Autodesk Inventor part; units mm, degrees
ref_plane "YZ Plane" through (0, 0, 0) normal (1, 0, 0) x (0, 1, 0)
ref_plane "XZ Plane" through (0, 0, 0) normal (0, 1, 0) x (-1, 0, 0)
ref_plane "XY Plane" through (0, 0, 0) normal (0, 0, 1) x (1, 0, 0)
sketch "Sketch1" plane through (0, 0, 0) normal (0, 0, 1) x (1, 0, 0)
  line L0 (0, 0) -> (24.765, 0)
  line L1 (24.765, 0) -> (24.765, 5.3594)
  line L2 (24.765, 5.3594) -> (0, 5.3594)
  line L3 (0, 5.3594) -> (0, 0)
  line L4 (23.7236, 7.3152) -> (30.734, 7.3152)
  line L5 (30.734, 7.3152) -> (30.734, 14.3256)
  line L6 (30.734, 14.3256) -> (23.7236, 14.3256)
  line L7 (23.7236, 14.3256) -> (23.7236, 7.3152)
  arc A0 (23.7236, 8.9916) -> (17.4244, 5.3594) centre (23.7236, 1.7133) ccw
  line L8 (24.765, 5.3594) -> (24.765, 7.3152)
  dimension "d0" = 24.765
  dimension "d1" = 5.3594
  dimension "d2" = 30.734
  dimension "d3" = 7.0104
  dimension "d4" = 14.3256
  dimension "d5" = 17.4244
  dimension "d6" = 5.334
extrude "Extrusion1" add sketch "Sketch1" along normal blind 25.4
fillet "Fillet1" radius 1.27 1 edges at (30.734, 14.3256, 12.7)
fillet "Fillet2" radius 1.27 2 edges at (30.734, 7.3152, 12.7) (23.7236, 14.3256, 12.7)
fillet "Fillet3" radius 1.27 5 edges at (23.7236, 8.9916, 12.7) (24.765, 7.3152, 12.7) (24.765, 0, 12.7) (0, 0, 12.7) (0, 5.3594, 12.7)
properties part number "Igus Slider"
The listing builds one solid part. Answer for the finished solid, in the listing's coordinates (mm). A direction names the side the tool comes from. Coordinates: 2 decimals unless noted, no trailing zeros. Loops run counter-clockwise (first coordinate to the right, second up) from the corner with the lowest first, then second, coordinate; pieces in that order, holes last.
1) Flat-ended cylindrical pins translate along their axes: pin 1 Ø2.5 at (y, z) = (3, 9.5) entering from +X (3 decimals); pin 2 Ø3 at (x, y) = (11, 8.5) entering from -Z; pin 3 Ø3 at (x, z) = (23, 19.5) entering from +Y; pin 4 Ø13 at (x, z) = (6, 9) entering from +Y. Find the tip coordinate at first contact, or state that the pin passes through.
2) Find section C-C on y = 11.25. Write down the section's boundary in (x, z), then the cut area to 3 significant figures.
3) Find section A-A on z = 12.25. Write down the section's boundary in (x, y) (3 decimals).
4) Find the intervals of material crossed by L1, parallel to X at y = 12.25, z = 20.5; L2, parallel to Y at x = 29.5, z = 16.25; L3, parallel to Y at x = 12, z = 18.75, in increasing order.
5) Find section B-B on x = 12.5. Write down the section's boundary in (y, z), then the cut area to 3 significant figures.
6) A tool of negligible diameter and unlimited length cuts with its end or side. For faces 1 (the face through (9, 5.359, 13)), 2 (the face through (24.765, 4, 13)), 3 (the face through (15, 4, 25.4)), from which of +Z, -Z, +X, -X, +Y, -Y can it reach the whole face along a straight path? Write none if from no direction.
Values:
1. pin 1: stops at x = 24.765
1. pin 2: passes through
1. pin 3: stops at y = 14.23
1. pin 4: stops at y = 5.36
2. outline: (23.72, 0) - (30.73, 0) - (30.73, 25.4) - (23.72, 25.4) - close
2. area: 178 mm2
3. outline: (0, 1.27) arc R1.27 ccw to (1.27, 0) - (23.495, 0) arc R1.27 ccw to (24.765, 1.27) - (24.765, 6.045) arc R1.27 cw to (26.035, 7.315) - (29.464, 7.315) arc R1.27 ccw to (30.734, 8.585) - (30.734, 13.056) arc R1.27 ccw to (29.464, 14.326) - (24.994, 14.326) arc R1.27 ccw to (23.724, 13.056) - (23.724, 10.167) arc R1.27 cw to (22.642, 8.911) arc R7.278 ccw to (17.424, 5.359) - (1.27, 5.359) arc R1.27 ccw to (0, 4.089) - close
4. L1: x = 23.72 to 30.73
4. L2: y = 7.32 to 14.33
4. L3: y = 0 to 5.36
5. outline: (0, 0) - (5.36, 0) - (5.36, 25.4) - (0, 25.4) - close
5. area: 136 mm2
6. face 1: +Z, -Z, -X, +Y
6. face 2: +Z, -Z, +X, -Y
6. face 3: +Z, +X, -X, +Y, -Y
